Geometry check sheet. Reference: the model listing, model coordinates, mm. Face numbers are marked on the shaded views. A direction names the side the tool comes from. Coordinates: 2 decimals unless noted, no trailing zeros. Write each loop counter-clockwise with the first axis right and the second up, starting at its lowest first coordinate (ties: lowest second). Pieces come first, ordered by that corner, then holes. Notation, with made-up numbers: (53, 26.25) -> (106, 26.25) arc R15 cw to (106, 30.25) -> close; hole circle Ø7 at (19.25, 56.5). An arc over 180 degrees is marked (long way). One line per question, with ' | ' between items.
from build123d import *

# Parameters (mm, degrees)
CUT_EXTRUDE1_REACH = 50.053
SKETCH2_R          = 7.5
FILLET1_R          = 3


with BuildPart() as part:
    # Sketch1 → Revolve1 (revolve)
    with BuildSketch(Plane(origin=(0, 0, 0), x_dir=(1, 0, 0), z_dir=(0, 1, 0))):
        with BuildLine():
            Line((0, 18.052635051), (0, 0))
            ThreePointArc((0, 0), (-14.509548929, 0.263245385), (-29, 1.052635051))
            Line((-29, 1.052635051), (-29, 18.052635051))
            Line((-29, 18.052635051), (-23.44, 18.052635051))
            Line((-23.44, 18.052635051), (-23.44, 21.052635051))
            Line((-23.44, 21.052635051), (-11.5, 21.052635051))
            Line((-11.5, 21.052635051), (-11.5, 48.052635051))
            Line((-11.5, 48.052635051), (-6, 48.052635051))
            Line((-6, 48.052635051), (-6, 18.052635051))
            Line((-6, 18.052635051), (0, 18.052635051))
        make_face()
    revolve(axis=Axis((0, 0, -358.843484937), (0, 0, 1)))

    # Sketch2 → Cut-Extrude1 (cut, up to next)
    with BuildSketch(Plane.XY, mode=Mode.PRIVATE) as cut_extrude1_sk1:
        with Locations((0, 29)):
            Circle(SKETCH2_R)
    cut_extrude1_tool1 = extrude(cut_extrude1_sk1.sketch, amount=-CUT_EXTRUDE1_REACH, mode=Mode.PRIVATE) & part.part
    add(cut_extrude1_tool1.solids().sort_by_distance((0, 29, 0))[0], mode=Mode.SUBTRACT)
    # Sketch2 → Cut-Extrude1 (cut, up to next)
    with BuildSketch(Plane.XY, mode=Mode.PRIVATE) as cut_extrude1_sk2:
        with Locations((29, 0)):
            Circle(SKETCH2_R)
    cut_extrude1_tool2 = extrude(cut_extrude1_sk2.sketch, amount=-CUT_EXTRUDE1_REACH, mode=Mode.PRIVATE) & part.part
    add(cut_extrude1_tool2.solids().sort_by_distance((29, 0, 0))[0], mode=Mode.SUBTRACT)
    # Sketch2 → Cut-Extrude1 (cut, up to next)
    with BuildSketch(Plane.XY, mode=Mode.PRIVATE) as cut_extrude1_sk3:
        with Locations((0, -29)):
            Circle(SKETCH2_R)
    cut_extrude1_tool3 = extrude(cut_extrude1_sk3.sketch, amount=-CUT_EXTRUDE1_REACH, mode=Mode.PRIVATE) & part.part
    add(cut_extrude1_tool3.solids().sort_by_distance((0, -29, 0))[0], mode=Mode.SUBTRACT)
    # Sketch2 → Cut-Extrude1 (cut, up to next)
    with BuildSketch(Plane.XY, mode=Mode.PRIVATE) as cut_extrude1_sk4:
        with Locations((-29, 0)):
            Circle(SKETCH2_R)
    cut_extrude1_tool4 = extrude(cut_extrude1_sk4.sketch, amount=-CUT_EXTRUDE1_REACH, mode=Mode.PRIVATE) & part.part
    add(cut_extrude1_tool4.solids().sort_by_distance((-29, 0, 0))[0], mode=Mode.SUBTRACT)

    # Fillet1
    fillet1_edges = [part.edges().sort_by_distance(p)[0] for p in [
        (-28.030172414, -7.437031293, -9.552634751),
        (-28.030172414, 7.437031293, -9.552635051),
        (7.437031293, -28.030172414, -9.552635051),
        (-7.437031293, -28.030172414, -9.552635051),
        (28.030172414, 7.437031293, -9.552635051),
        (28.030172414, -7.437031293, -9.552635051),
        (-7.437031293, 28.030172414, -9.552635051),
        (7.437031293, 28.030172414, -9.552635051),
    ]]
    fillet(fillet1_edges, radius=FILLET1_R)


solid = part.part
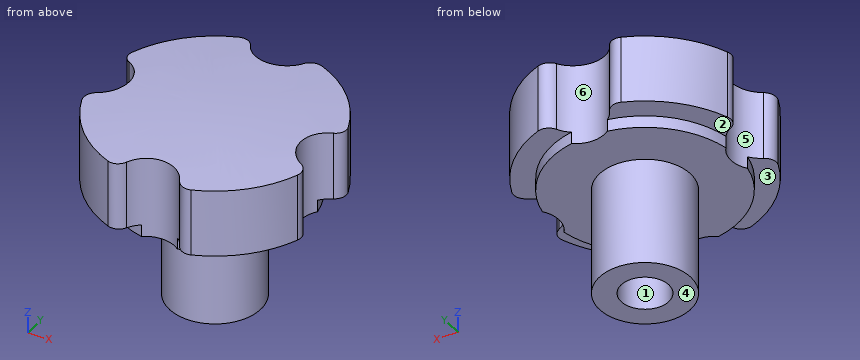
1. Cross-section at D-D on x = -18. Record the boundary of the cut face in (y, z), and give its area (3 significant figures).
Worked answers:
outline: (-22.74, -18.05) -> (-15.01, -18.05) -> (-15.01, -21.05) -> (15.01, -21.05) -> (15.01, -18.05) -> (22.74, -18.05) -> (22.74, -1.05) arc R399.59 ccw to (-22.74, -1.05) -> close | area: 883 mm²
2. Cross-section at A-A on x = 0. Record the boundary of the cut face in (y, z), and give its area (3 significant figures).
Worked answers:
outline: (-21.5, -21.05) -> (-11.5, -21.05) -> (-11.5, -48.05) -> (-6, -48.05) -> (-6, -18.05) -> (6, -18.05) -> (6, -48.05) -> (11.5, -48.05) -> (11.5, -21.05) -> (21.5, -21.05) -> (21.5, -0.58) arc R400 ccw to (-21.5, -0.58) -> close | area: 1,160 mm²
3. Mould release check, pull along Y, two halves, no side actions. Record for the marked faces 4, 5 and 6: released by +Y, released by -Y, zero draft, split by the parting line, or undercut.
Worked answers:
face 4: zero draft | face 5: undercut | face 6: released by +Y
4. Material ranges on line 1 (X direction, y = 0, z = -31.5); line 2 (X direction, y = -22.5, z = -14), recorded low to high. Write a range as from..to.
Worked answers:
line 1: -11.5..-6, 6..11.5 | line 2: -18.3..-3.74, 3.74..18.3
5. Cross-section at C-C on z = -42. Record the boundary of the cut face in (x, y), and give its area (3 significant figures).
Worked answers:
outline: circle Ø23 at (0, 0); hole circle Ø12 at (0, 0) | area: 302 mm²
6. Go/stop test with flat-tipped pins: P1, Ø1.5, axis at x = 10, z = -39, coming from the -Y side; P2, Ø6, axis at x = 21, y = -21.5, coming from the +Z side; P3, Ø3, axis at x = -12, z = -37.5, coming from the +Y side; P4, Ø7, axis at x = 0, y = 0, coming from the +Z side. Record where each tip stops, or that it passes through.
Worked answers:
P1: y = -6.83 | P2: z = -0.92 | P3: y = 4.69 | P4: z = 0
7. Tool access check on the marked faces 1, 2 and 3. Record the directions out of +Z, -Z, +X, -X, +Y, -Y that give a thin tool (end or side, any length) a straight path to the whole face; none if there is none.
Worked answers:
face 1: -Z | face 2: -Z, -X, +Y | face 3: -Z, -X, -Y
